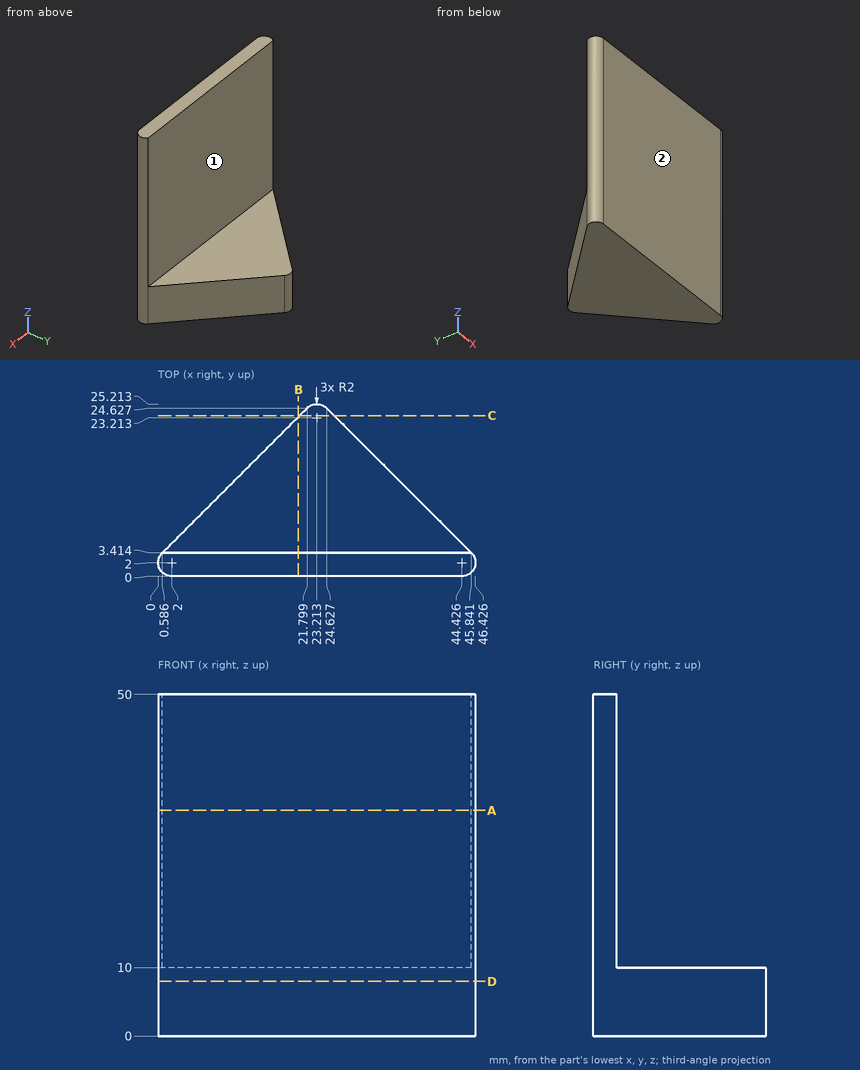
For this review, use the dimensioned drawing (mm, ordinates from the lowest corner) and the shaded views. A direction names the side the tool comes from. Round coordinates to 2 decimals unless told otherwise and drop trailing zeros. Order: outer loops, then holes, each group sorted by start corner. A loop starts at its lowest first (then second) coordinate and runs counter-clockwise, first axis right, second up. Notation, with made-up numbers: M 12,88 L 28,88 A16 ccw 28,119 Z; hole C 62,16.25 d6. An arc over 180 degrees is marked long. Use a Markdown table: item, result. Add a question column.
Item 1: Tool access review of the marked faces 1 and 2: name each direction out of +Z, -Z, +X, -X, +Y, -Y from which nothing blocks a thin tool from reaching the whole face with its end or side.
Item 2: To check wall thickness, follow line 1 along Y through (x, z) = (21, 35) (1 decimal); line 2 along Z through (x, y) = (28, 20); line 3 along X through (y, z) = (11.5, 7.5) (1 decimal). State the ranges of each line that lie inside material, in increasing order.
Item 3: Insertion check: pin 1 (1.5 mm diameter, centred on x = 32, y = 15.5, fed in from +Z); pin 2 (20 mm diameter, centred on x = 29, z = 27, fed in from +Y); pin 3 (1 mm diameter, centred on y = 16, z = 6.5, fed in from -X). Each pin has a flat end and moves straight along its axis. Give the tip position at first contact, or say it passes through.
Item 4: Add section A-A, the plane z = 33. Give the boundary of the cut face in (x, y) (1 decimal).
Item 5: Add section D-D, the plane z = 8. Give the boundary of the cut face in (x, y) (1 decimal).
Item 6: Add section C-C, the plane y = 23.5. Give the boundary of the cut face in (x, z) (1 decimal).
Item 7: Add section B-B, the plane x = 20.5. Give the boundary of the cut face in (y, z) (1 decimal), then the cut area to 3 significant figures.
Geometry results:
| question | item | result |
|---|---|---|
| 1 | face 1 | +Z, +X, -X, +Y |
| 1 | face 2 | +Z, -Z, +X, -X, -Y |
| 2 | line 1 | y = 0 to 3.4 |
| 2 | line 2 | z = 0 to 10 |
| 2 | line 3 | x = 8.7 to 37.8 |
| 3 | pin 1 | stops at z = 10 |
| 3 | pin 2 | stops at y = 3.41 |
| 3 | pin 3 | stops at x = 12.67 |
| 4 | outline | M 0.6,3.4 A2 ccw 2,0 L 44.4,0 A2 ccw 45.8,3.4 Z |
| 5 | outline | M 0.6,3.4 A2 ccw 2,0 L 44.4,0 A2 ccw 45.8,3.4 L 24.6,24.6 A2 ccw 21.8,24.6 Z |
| 6 | outline | M 20.7,0 L 25.8,0 L 25.8,10 L 20.7,10 Z |
| 7 | outline | M 0,0 L 23.3,0 L 23.3,10 L 3.4,10 L 3.4,50 L 0,50 Z |
| 7 | area | 370 mm² |
